Geometry: see drawing. Coordinates: mm, zero at the bounding-box minimum. A direction names the side the tool comes from. Round coordinates to 2 decimals unless told otherwise and drop trailing zeros. Order: outer loops, then holes, each group sorted by start corner. A loop starts at its lowest first (then second) coordinate and runs counter-clockwise, first axis right, second up. Notation, with made-up numbers: M -5,58.25 L 53,58.25 A16 cw 53,67.25 Z; hole C 12,73 d11. An arc over 180 degrees is marked long. Answer in a Markdown table with one row per item. Add a question column.
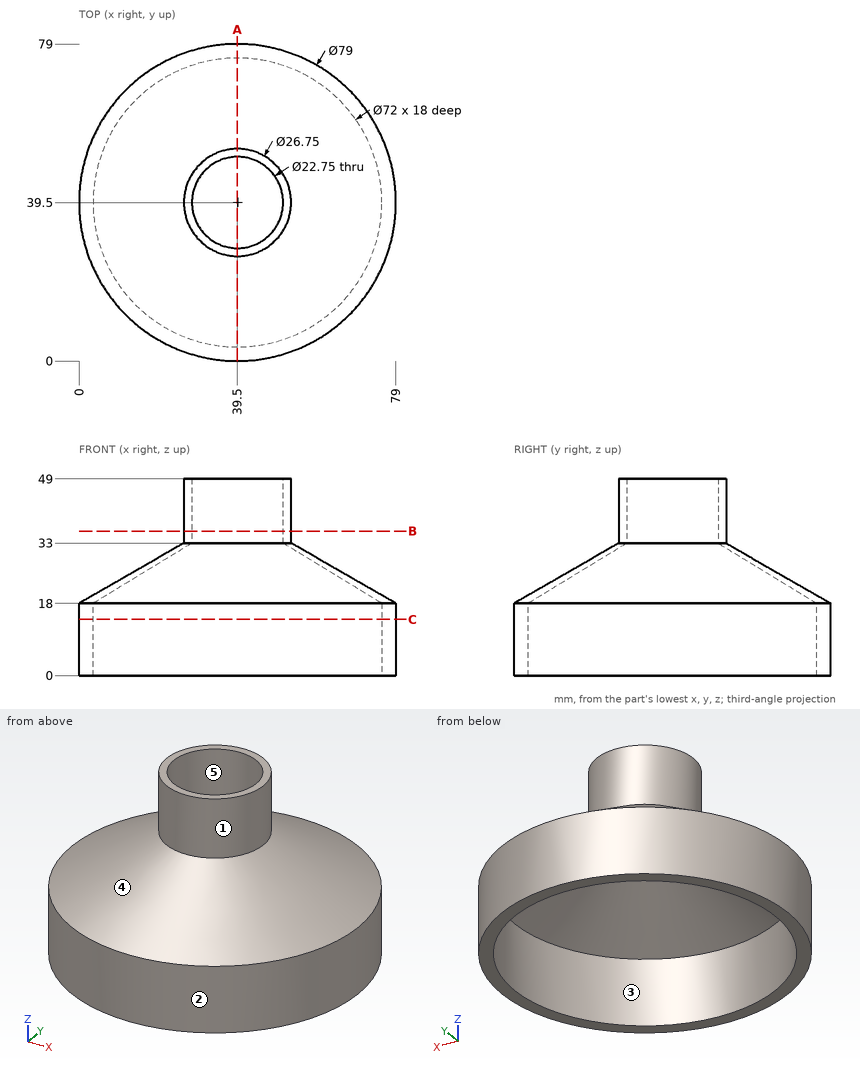
(1) Draft query along X for the marked faces 4 and 5. Return one class per face: +X half, -X half, draft (parallel to the pull), parting line (faces both ways), or undercut.
(2) Access query for the marked faces 1, 2 and 3. Directions: +Z, -Z, +X, -X, +Y, -Y. A direction counts if a zero-diameter tool reaches every point of the face in a straight line with its end or side. Return the directions, or none.
(3) Cut plane B-B (z = 36). Return loops of the section in (x, y) (3 decimals), and give its area (3 significant figures).
(4) Cut plane C-C (z = 14). Return loops of the section in (x, y).
(5) Pin query (flat end, axial travel): pin 1 (1 mm diameter, centred on x = 29, z = 11, fed in from -Y); pin 2 (4 mm diameter, centred on y = 47.5, z = 11, fed in from +X); pin 3 (1.5 mm diameter, centred on x = 69.5, z = 18, fed in from -Y); pin 4 (5 mm diameter, centred on y = 40, z = 19, fed in from -X). Return the tip coordinate at first contact, or that it passes through.
(6) Line query: line 1 (Y direction, x = 39.5, z = 38) (3 decimals); line 2 (Y direction, x = 39.5, z = 7.5). Output: solid intervals per line, ascending. Write a range as from..to.
(7) Cut plane A-A (x = 39.5). Return loops of the section in (y, z) (3 decimals).
Answer list:
| question | item | result |
|---|---|---|
| 1 | face 4 | parting line |
| 1 | face 5 | undercut |
| 2 | face 1 | +Z |
| 2 | face 2 | +Z, -Z |
| 2 | face 3 | -Z |
| 3 | outline | C 39.5,39.5 d26.75; hole C 39.5,39.5 d22.75 |
| 3 | area | 156 mm² |
| 4 | outline | C 39.5,39.5 d79; hole C 39.5,39.5 d72 |
| 5 | pin 1 | y = 1.29 |
| 5 | pin 2 | x = 78.54 |
| 5 | pin 3 | y = 12.95 |
| 5 | pin 4 | x = 0 |
| 6 | line 1 | 26.125..28.125, 50.875..52.875 |
| 6 | line 2 | 0..3.5, 75.5..79 |
| 7 | outline | M 0,0 L 3.5,0 L 3.5,18 L 28.125,33 L 28.125,49 L 26.125,49 L 26.125,33 L 0,18 Z; M 50.875,33 L 75.5,18 L 75.5,0 L 79,0 L 79,18 L 52.875,33 L 52.875,49 L 50.875,49 Z |
